Part model, mm, in its own coordinate system. Round coordinates to 2 decimals unless told otherwise and drop trailing zeros. Loops run counter-clockwise (first coordinate to the right, second up) from the corner with the lowest first, then second, coordinate; pieces in that order, holes last. Notation, with made-up numbers: (64, -21.75) -> (72, -21.75) arc R20 cw to (72, -15.75) -> close; hole circle Ø10 at (46, 17). An arc over 180 degrees is marked (long way). Answer as a JSON object with one key per item and string values. Group by question number.
from build123d import *

# Parameters (mm, degrees)
SKETCH1_W           = 382.452818204
SKETCH1_H           = 50.8
SKETCH1_R           = 14.3002
SKETCH1_R_2         = 2.54
BOSS_EXTRUDE1_DEPTH = 3.175
FILLET1_R           = 7.62


with BuildPart() as part:
    # Sketch1 → Boss-Extrude1 (new body)
    with BuildSketch(Plane.XY):
        with Locations((132.2654537, 9.352736133)):
            Rectangle(SKETCH1_W, SKETCH1_H)
        with Locations((-34.334788468, 9.352736133)):
            Circle(SKETCH1_R, mode=Mode.SUBTRACT)
        with Locations((298.913211532, 9.352736133)):
            Circle(SKETCH1_R, mode=Mode.SUBTRACT)
        with Locations((53.803211532, 9.352736133)):
            Circle(SKETCH1_R, mode=Mode.SUBTRACT)
        with Locations((87.573397818, 9.352736133)):
            Circle(SKETCH1_R, mode=Mode.SUBTRACT)
        with Locations((19.729570927, 9.352736133)):
            Circle(SKETCH1_R, mode=Mode.SUBTRACT)
        with Locations((156.877176863, 9.352736133)):
            Circle(SKETCH1_R_2, mode=Mode.SUBTRACT)
        with Locations((169.577176863, 9.352736133)):
            Circle(SKETCH1_R_2, mode=Mode.SUBTRACT)
        with Locations((182.277176863, 9.352736133)):
            Circle(SKETCH1_R_2, mode=Mode.SUBTRACT)
        with Locations((194.977176863, 9.352736133)):
            Circle(SKETCH1_R_2, mode=Mode.SUBTRACT)
        with Locations((207.677176863, 9.352736133)):
            Circle(SKETCH1_R_2, mode=Mode.SUBTRACT)
        with Locations((-2.968643943, 28.669348732)):
            Circle(SKETCH1_R_2, mode=Mode.SUBTRACT)
        with Locations((9.731356057, 28.669348732)):
            Circle(SKETCH1_R_2, mode=Mode.SUBTRACT)
        with Locations((22.431356057, 28.669348732)):
            Circle(SKETCH1_R_2, mode=Mode.SUBTRACT)
        with Locations((35.131356057, 28.669348732)):
            Circle(SKETCH1_R_2, mode=Mode.SUBTRACT)
        with Locations((47.831356057, 28.669348732)):
            Circle(SKETCH1_R_2, mode=Mode.SUBTRACT)
        with Locations((60.531356057, 28.669348732)):
            Circle(SKETCH1_R_2, mode=Mode.SUBTRACT)
        with Locations((73.231356057, 28.669348732)):
            Circle(SKETCH1_R_2, mode=Mode.SUBTRACT)
        with Locations((85.931356057, 28.669348732)):
            Circle(SKETCH1_R_2, mode=Mode.SUBTRACT)
        with Locations((98.631356057, 28.669348732)):
            Circle(SKETCH1_R_2, mode=Mode.SUBTRACT)
        with Locations((111.331356057, 28.669348732)):
            Circle(SKETCH1_R_2, mode=Mode.SUBTRACT)
        with Locations((111.331356057, 15.969348732)):
            Circle(SKETCH1_R_2, mode=Mode.SUBTRACT)
        with Locations((111.331356057, 3.269348732)):
            Circle(SKETCH1_R_2, mode=Mode.SUBTRACT)
        with Locations((9.731356057, -9.430651268)):
            Circle(SKETCH1_R_2, mode=Mode.SUBTRACT)
        with Locations((22.431356057, -9.430651268)):
            Circle(SKETCH1_R_2, mode=Mode.SUBTRACT)
        with Locations((35.131356057, -9.430651268)):
            Circle(SKETCH1_R_2, mode=Mode.SUBTRACT)
        with Locations((47.831356057, -9.430651268)):
            Circle(SKETCH1_R_2, mode=Mode.SUBTRACT)
        with Locations((60.531356057, -9.430651268)):
            Circle(SKETCH1_R_2, mode=Mode.SUBTRACT)
        with Locations((73.231356057, -9.430651268)):
            Circle(SKETCH1_R_2, mode=Mode.SUBTRACT)
        with Locations((85.931356057, -9.430651268)):
            Circle(SKETCH1_R_2, mode=Mode.SUBTRACT)
        with Locations((98.631356057, -9.430651268)):
            Circle(SKETCH1_R_2, mode=Mode.SUBTRACT)
        with Locations((111.331356057, -9.430651268)):
            Circle(SKETCH1_R_2, mode=Mode.SUBTRACT)
        with Locations((-2.968643943, 15.969348732)):
            Circle(SKETCH1_R_2, mode=Mode.SUBTRACT)
        with Locations((-2.968643943, 3.269348732)):
            Circle(SKETCH1_R_2, mode=Mode.SUBTRACT)
        with Locations((-2.968643943, -9.430651268)):
            Circle(SKETCH1_R_2, mode=Mode.SUBTRACT)
    extrude(amount=BOSS_EXTRUDE1_DEPTH)

    # Fillet1
    fillet1_edges = [part.edges().sort_by_distance(p)[0] for p in [
        (-58.960955402, 34.752736133, 1.5875),
        (323.491862802, 34.752736133, 1.5875),
        (323.491862802, -16.047263867, 1.5875),
        (-58.960955402, -16.047263867, 1.5875),
    ]]
    fillet(fillet1_edges, radius=FILLET1_R)


solid = part.part
Item 1: Two-plate mould, pull along X, no slides. Class faces 1 (the face through (130, 10, 3.175)), 2 (the face through (-56.788, -13.756, 1.61)), 3 (the face through (33.37, 13.65, 1.57)), 4 (the face through (321.2, 32.58, 1.61)): pulls with the +X half, pulls with the -X half, needs draft (parallel to the pull), parting line crosses it, or undercut.
Item 2: Band-saw the part on A-A, the plane x = -24. List the corners of the cut face in (y, z) (3 decimals).
Item 3: Band-saw the part on B-B, the plane z = 2.2. Count the separate pieces of the cut face and the enclosed holes in it, plus the area to 3 significant figures.
Item 4: Drop flat-ended pins along their axis: pin 1 Ø8 at (x, y) = (98.63, -9.43) entering from -Z; pin 2 Ø4.5 at (x, y) = (85.93, -9.43) entering from +Z. Give the stop position or say it passes through.
Item 5: Drill centre lines: line 1 (Y direction, x = 97.5, z = 2.6); line 2 (X direction, y = 20.5, z = 2.2); line 3 (Y direction, x = -34.5, z = 0.5). Where is each one in solid material? Low to high.
Entries:
{
 "1": {"face 1": "needs draft", "face 2": "pulls with the -X half", "face 3": "undercut", "face 4": "pulls with the +X half"},
 "2": {"outline": "(-16.047, 0) -> (-0.531, 0) -> (-0.531, 3.175) -> (-16.047, 3.175) -> close; (19.236, 0) -> (34.753, 0) -> (34.753, 3.175) -> (19.236, 3.175) -> close"},
 "3": {"separate pieces": "1", "enclosed holes": "34", "area": "15,600 mm²"},
 "4": {"pin 1": "z = 0", "pin 2": "through"},
 "5": {"line 1": "-16.05 to -11.7, -7.16 to -0.94, 19.65 to 26.4, 30.94 to 34.75", "line 2": "-58.96 to -43.29, -25.38 to 10.77, 28.69 to 44.85, 62.76 to 78.62, 96.53 to 289.96, 307.87 to 323.49", "line 3": "-16.05 to -4.95, 23.65 to 34.75"}
}
